```python
from build123d import *

# Parameters (mm, degrees)
SKETCH002_R   = 4
PAD002_DEPTH  = 18
SKETCH001_R   = 4
PAD001_DEPTH  = 18
SKETCH003_W   = 12.468703
SKETCH003_H   = 5.180136
SKETCH003_W_2 = 5.180136
SKETCH003_H_2 = 12.468704
PAD003_DEPTH  = 5
SKETCH004_W   = 4
SKETCH004_H   = 2
SKETCH004_W_2 = 2
SKETCH004_H_2 = 4
PAD004_DEPTH  = 2.5
SKETCH_R      = 4
PAD_DEPTH     = 10


with BuildPart() as mount002:
    # Sketch002 → Pad002 (new body)
    with BuildSketch(Plane.XZ.offset(-27)):
        with Locations((-1, 10)):
            Circle(SKETCH002_R)
    extrude(amount=PAD002_DEPTH)


with BuildPart() as mount001:
    # Sketch001 → Pad001 (new body)
    with BuildSketch(Plane.YZ.offset(27)):
        with Locations((-1, 10)):
            Circle(SKETCH001_R)
    extrude(amount=-PAD001_DEPTH)


with BuildPart() as cutblock:
    # Sketch003 → Pad003 (new body)
    with BuildSketch(Plane.XY.offset(10)):
        with Locations((-1.285158, 14.590068)):
            Rectangle(SKETCH003_W, SKETCH003_H)
        with Locations((14.590068, -0.774081)):
            Rectangle(SKETCH003_W_2, SKETCH003_H_2)
    extrude(amount=-PAD003_DEPTH)

    # Fusion001: union Mount002, Mount001
    add(mount002.part)
    add(mount001.part)


with BuildPart() as clip:
    # Sketch004 → Pad004 (new body)
    with BuildSketch(Plane.XY.offset(10)):
        with Locations((0, 6.5)):
            Rectangle(SKETCH004_W, SKETCH004_H)
        with Locations((6.5, 0)):
            Rectangle(SKETCH004_W_2, SKETCH004_H_2)
        Polygon((-6.717514, -3.889087), (-5.303301, -2.474874), (-2.474874, -5.303301), (-3.889087, -6.717514), align=None)
    extrude(amount=PAD004_DEPTH)


with BuildPart() as cut:
    # Sketch → Pad (new body)
    with BuildSketch(Plane.XY):
        with BuildLine():
            Line((-9, 3.6e-05), (-9, 27))
            Line((-9, 27), (7, 27))
            Line((7, 27), (7, 7))
            Line((7, 7), (27, 7))
            Line((27, 7), (27, -9))
            Line((27, -9), (3.6e-05, -9))
            ThreePointArc((-9, 3.6e-05), (-6.363961, -6.363961), (3.6e-05, -9))
        make_face()
        Circle(SKETCH_R, mode=Mode.SUBTRACT)
    extrude(amount=PAD_DEPTH)

    # Fusion: union Clip
    add(clip.part)

    # Cut: cut CutBlock
    add(cutblock.part, mode=Mode.SUBTRACT)


solid = cut.part
```
Here's how the part is built. I have some questions about the finished solid (model axes, mm). A direction names the side the tool comes from. Round coordinates to 2 decimals unless told otherwise and drop trailing zeros. Write each loop counter-clockwise with the first axis right and the second up, starting at its lowest first coordinate (ties: lowest second). Pieces come first, ordered by that corner, then holes.
Q1. If we section it at B-B on y = 3.5: Write out the boundary of the cut face in (x, z).
Q2. If we section it at C-C on x = -0.5: Write out the boundary of the cut face in (y, z), plus the area to 3 significant figures.
Q3. If we section it at D-D on y = 15: Write out the boundary of the cut face in (x, z).
Q4. If we mould it in two halves opening along X, with no side actions, what happens to faces 4 (the flat face through (-5, -5, 12.5)), 5 (the flat face through (-9, 13, 5)), 6 (the flat face through (-3, 12, 6)), 7 (the flat face through (-1, 9, 8))? For each: +X half, -X half, draft (parallel to the pull), parting line (faces both ways), or undercut.
Q5. Will these pins go through, and if not, where does the flat tip stop? P1, Ø2, axis at y = 1.5, z = 9, coming from the +X side; P2, Ø3, axis at x = -2, z = 9, coming from the +Y side; P3, Ø4, axis at x = -2.5, z = 8, coming from the -Y side.
Q6. Which directions (+Z, -Z, +X, -X, +Y, -Y) give clear straight access to the entire face, cutting with the end or side of a thin tool? Please do faces 1 (the flat face through (0, 5.5, 11)), 2 (the flat face through (7.5, 0, 11)), 3 (the flat face through (0, 7.5, 11)).
Q7. Please list where these lines run through material, in increasing order: probe 1 along Y at (x, z) = (0, 6.5); probe 2 along Y at (x, z) = (15.5, 7.5); probe 3 along Z at (x, y) = (3, -6).
Q8. If we section it at A-A on z = 3.75: Write out the boundary of the cut face in (x, y), plus the area to 3 significant figures.
Answer below:
1. outline: (-9, 0) - (-1.94, 0) - (-1.94, 10) - (-9, 10) - close; (1.94, 0) - (27, 0) - (27, 10) - (17.18, 10) - (17.18, 5) - (12, 5) - (12, 10) - (1.94, 10) - close
2. outline: (-8.99, 0) - (-3.97, 0) - (-3.97, 10) - (-8.99, 10) - close; (3.97, 0) - (27, 0) - (27, 6.03) - (17.18, 6.03) - (17.18, 5) - (12, 5) - (12, 6.03) - (9, 6.03) - (9, 10) - (7.5, 10) - (7.5, 12.5) - (5.5, 12.5) - (5.5, 10) - (3.97, 10) - close
2. area: 209 mm2
3. outline: (-9, 0) - (7, 0) - (7, 10) - (4.95, 10) - (4.95, 5) - (-7.52, 5) - (-7.52, 10) - (-9, 10) - close
4. face 4: draft
4. face 5: -X half
4. face 6: undercut
4. face 7: undercut
5. P1: stops at x = 9
5. P2: stops at y = 9
5. P3: stops at y = -8.99
6. face 1: +Z, +X, -X, -Y
6. face 2: +Z, +X, +Y, -Y
6. face 3: +Z, +X, -X, +Y
7. probe 1: y = -9 to -4, 4 to 9
7. probe 2: y = -9 to -7.01, 5.46 to 7
7. probe 3: z = 0 to 10
8. outline: (-9, 0) arc R9 ccw to (0, -9) - (27, -9) - (27, 7) - (7, 7) - (7, 27) - (-9, 27) - close; hole circle Ø8 at (0, 0)
8. area: 828 mm2
